Design review of the part built by this model. Coordinates are the model's own, in mm. A direction names the side the tool comes from. Coordinates: 2 decimals unless noted, no trailing zeros. One line per item, written item: value.
Autodesk Inventor part; units mm, degrees
ref_plane "YZ Plane" through (0, 0, 0) normal (1, 0, 0) x (0, 1, 0)
ref_plane "XZ Plane" through (0, 0, 0) normal (0, 1, 0) x (-1, 0, 0)
ref_plane "XY Plane" through (0, 0, 0) normal (0, 0, 1) x (1, 0, 0)
sketch "Sketch1" plane through (0, 0, 0) normal (0, 0, 1) x (1, 0, 0)
  line L0 (-10, 0) -> (-10, 5)
  line L1 (-10, 5) -> (10, 5)
  line L2 (10, 5) -> (10, 0)
  line L3 (10, 0) -> (-10, 0)
  line L4 (-9.5, 5) -> (-8.5, 5)
  line L5 (-8.5, 5) -> (-8.5, 6)
  line L6 (-8.5, 6) -> (-9.5, 6)
  line L7 (-9.5, 6) -> (-9.5, 5)
  line L8 (-6.5, 5) -> (-6.5, 6)
  line L9 (-7.5, 6) -> (-7.5, 5)
  line L10 (-6.5, 6) -> (-7.5, 6)
  line L11 (-4.5, 5) -> (-4.5, 6)
  line L12 (-5.5, 6) -> (-5.5, 5)
  line L13 (-4.5, 6) -> (-5.5, 6)
  line L14 (-2.5, 5) -> (-2.5, 6)
  line L15 (-3.5, 6) -> (-3.5, 5)
  line L16 (-2.5, 6) -> (-3.5, 6)
  line L17 (-0.5, 5) -> (-0.5, 6)
  line L18 (-1.5, 6) -> (-1.5, 5)
  line L19 (-0.5, 6) -> (-1.5, 6)
  line L20 (1.5, 5) -> (1.5, 6)
  line L21 (0.5, 6) -> (0.5, 5)
  line L22 (1.5, 6) -> (0.5, 6)
  line L23 (3.5, 5) -> (3.5, 6)
  line L24 (2.5, 6) -> (2.5, 5)
  line L25 (3.5, 6) -> (2.5, 6)
  line L26 (5.5, 5) -> (5.5, 6)
  line L27 (4.5, 6) -> (4.5, 5)
  line L28 (5.5, 6) -> (4.5, 6)
  line L29 (7.5, 5) -> (7.5, 6)
  line L30 (6.5, 6) -> (6.5, 5)
  line L31 (7.5, 6) -> (6.5, 6)
  line L32 (9.5, 5) -> (9.5, 6)
  line L33 (8.5, 6) -> (8.5, 5)
  line L34 (9.5, 6) -> (8.5, 6)
  point P0 (0, 0)
  point P1 (0, -80)
  dimension "d0" = 5
  dimension "d1" = 20
  dimension "d2" = 90
  dimension "d10" = 1
  dimension "d11" = 1
  dimension "d14" = 2
sketch "Sketch2" plane through (0, 0, 0) normal (0, 0, 1) x (1, 0, 0)
  line L0 (0, -80.0206) -> (52.1093, -80.0206) construction
  point P0 (0, 0)
revolve "Revolution1" add sketch "Sketch1" angle 360 about axis through (0, -80.0206, 0) along (1, 0, 0)
properties part number "TPU Tire"
1. Mouldability with a two-part tool opening along Z and no side actions: class faces 5 (the face through (-0.14, -6.102, 30.648)), 6 (the face through (-1.5, -100, 83)), 7 (the face through (6.01, -40.79, -75.43)) as released by +Z, released by -Z, zero draft, split by the parting line, or undercut.
Answer block:
face 5: undercut
face 6: zero draft
face 7: split by the parting line
2. Wall thickness on line 1 along Z through (x, y) = (-3.25, -129.5); line 2 along Y through (x, z) = (0, 23.5); line 3 along Y through (x, z) = (-4.25, -22): over which ranges is each line inside the solid? List them lowest first.
Answer block:
line 1: z = -70.37 to -62.89, 62.89 to 70.37
line 2: y = -161.73 to -156.51, -3.53 to 1.69
line 3: y = -162.15 to -156.96, -3.08 to 2.1
3. For faces 1 (the face through (-9.75, -40.79, -75.43)), 2 (the face through (8.5, -100, 83)), 3 (the face through (-1.01, -165.96, -3.78)), 4 (the face through (9.5, -100, 83)), list the 3-axis set-ups (+Z, -Z, +X, -X, +Y, -Y) from which the entire face can be reached by the end or side of a thin tool; tool diameter is ignored.
Answer block:
face 1: -X
face 2: none
face 3: +X, -X
face 4: +X
4. Insertion check: pin 1 Ø2 at (x, z) = (-7.5, -41) entering from -Y; pin 2 Ø2 at (x, z) = (7, 60.5) entering from +Y; pin 3 Ø5 at (x, y) = (2.5, -49.5) entering from -Z. Each pin has a flat end and moves straight along its axis. Give the tip position at first contact, or say it passes through.
Answer block:
pin 1: stops at y = -156.18
pin 2: stops at y = -17.9
pin 3: stops at z = -81.33
